from build123d import *

# Parameters (mm, degrees)
SKETCH1_W           = 400
SKETCH1_H           = 80
BOSS_EXTRUDE1_DEPTH = 20
SKETCH5_W           = 400
SKETCH5_H           = 10
BOSS_EXTRUDE2_DEPTH = 30
SKETCH7_W           = 400
SKETCH7_H           = 10
BOSS_EXTRUDE3_DEPTH = 30
BOSS_EXTRUDE4_START = -20
SKETCH8_W           = 100
SKETCH8_H           = 60
BOSS_EXTRUDE4_DEPTH = 490
SKETCH9_W           = 80
SKETCH9_H           = 50
CUT_EXTRUDE1_DEPTH  = 940
SKETCH11_W          = 80
SKETCH11_H          = 50
BOSS_EXTRUDE5_DEPTH = 20
MIRROR20_START      = -30
MIRROR20_OUTLINE_W  = 490
MIRROR20_OUTLINE_H  = 100
MIRROR20_DEPTH      = 60
SKETCH12_R          = 15
CUT_EXTRUDE2_DEPTH  = 1031.388276331
SKETCH19_R          = 15
CUT_EXTRUDE10_DEPTH = 1031.388276331


# Read off the part's stored shape, not the designer's step: Mirror20
with BuildPart() as part:
    # Sketch1 → Boss-Extrude1 (new body)
    with BuildSketch(Plane(origin=(0, 0, 0), x_dir=(0, 0, -1), z_dir=(1, 0, 0))):
        Rectangle(SKETCH1_W, SKETCH1_H)
    boss_extrude1 = extrude(amount=BOSS_EXTRUDE1_DEPTH)

    # Sketch5 → Boss-Extrude2 (add)
    with BuildSketch(Plane.ZY):
        with Locations((0, 35)):
            Rectangle(SKETCH5_W, SKETCH5_H)
    boss_extrude2 = extrude(amount=BOSS_EXTRUDE2_DEPTH)

    # Sketch7 → Boss-Extrude3 (add)
    with BuildSketch(Plane(origin=(20, 0, 0), x_dir=(0, 0, -1), z_dir=(1, 0, 0))):
        with Locations((0, -35)):
            Rectangle(SKETCH7_W, SKETCH7_H)
    boss_extrude3 = extrude(amount=BOSS_EXTRUDE3_DEPTH)

    # Sketch8 → Boss-Extrude4 (add)
    with BuildSketch(Plane.ZY.offset(BOSS_EXTRUDE4_START)):
        Rectangle(SKETCH8_W, SKETCH8_H)
    extrude(amount=BOSS_EXTRUDE4_DEPTH)

    # Sketch9 → Cut-Extrude1 (cut)
    with BuildSketch(Plane.ZY.offset(470)):
        with Locations((0, -5)):
            Rectangle(SKETCH9_W, SKETCH9_H)
    cut_extrude1 = extrude(amount=-CUT_EXTRUDE1_DEPTH, mode=Mode.SUBTRACT)

    # Sketch11 → Boss-Extrude5 (add)
    with BuildSketch(Plane(origin=(20, 0, 0), x_dir=(0, 0, -1), z_dir=(1, 0, 0))):
        with Locations((0, -5)):
            Rectangle(SKETCH11_W, SKETCH11_H)
    boss_extrude5 = extrude(amount=-BOSS_EXTRUDE5_DEPTH)

    # Mirror20 outline → Mirror20 (add)
    with BuildSketch(Plane(origin=(0, 0, 0), x_dir=(1, 0, 0), z_dir=(0, 1, 0)).offset(MIRROR20_START)):
        with Locations((-715, 0)):
            Rectangle(MIRROR20_OUTLINE_W, MIRROR20_OUTLINE_H)
    extrude(amount=MIRROR20_DEPTH)

    # Mirror22: Boss-Extrude1, Boss-Extrude2, Boss-Extrude3, Cut-Extrude1, Boss-Extrude5 across plane
    add(boss_extrude1.mirror(Plane.ZY.offset(470)))
    add(boss_extrude2.mirror(Plane.ZY.offset(470)))
    add(boss_extrude3.mirror(Plane.ZY.offset(470)))
    add(cut_extrude1.mirror(Plane.ZY.offset(470)), mode=Mode.SUBTRACT)
    add(boss_extrude5.mirror(Plane.ZY.offset(470)))

    # Sketch12 → Cut-Extrude2 (cut, through all)
    with BuildSketch(Plane.ZY.offset(960)):
        with Locations((89.62, 0)):
            Circle(SKETCH12_R)
    extrude(amount=-CUT_EXTRUDE2_DEPTH, mode=Mode.SUBTRACT)

    # Sketch19 → Cut-Extrude10 (cut, through all)
    with BuildSketch(Plane.ZY.offset(960)):
        with Locations((-128.216, 0)):
            Circle(SKETCH19_R)
    extrude(amount=-CUT_EXTRUDE10_DEPTH, mode=Mode.SUBTRACT)


solid = part.part
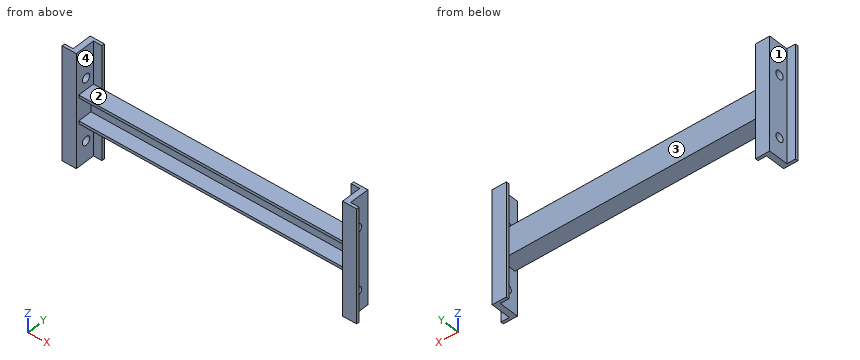
Work out the finished part from the listing and answer in its coordinate system (mm). Face numbers are marked on the shaded views. A direction names the side the tool comes from. Give positions to 0.01 mm unless a question says otherwise; leave off trailing zeros. Loops run counter-clockwise (first coordinate to the right, second up) from the corner with the lowest first, then second, coordinate; pieces in that order, holes last. Notation, with made-up numbers: (22.25, 53.5) -> (49.25, 53.5) arc R17 cw to (49.25, 72.5) -> close; hole circle Ø4 at (7, 52.25). An arc over 180 degrees is marked (long way). Use a Markdown table: item, result. Add a question column.
1. Flat-ended cylindrical pins translate along their axes: pin 1 Ø15 at (x, z) = (-977.5, -50) entering from +Y; pin 2 Ø2 at (y, z) = (-27, -24) entering from +X; pin 3 Ø4 at (x, z) = (-586.5, -47) entering from -Y; pin 4 Ø24 at (y, z) = (0, -128.216) entering from +X (3 decimals). Find the tip coordinate at first contact, or state that the pin passes through.
2. For the marked faces 3 and 4, determine the directions among +Z, -Z, +X, -X, +Y, -Y from which every point of the face is accessible in a straight line to the end or side of a thin tool.
3. Section C-C on x = -456 is taken. Determine the outline of the cut face in (y, z), and give its area (3 significant figures).
4. Find the intervals of material crossed by probe 1 along X at (y, z) = (-26, 67); probe 2 along X at (y, z) = (-30.5, -42); probe 3 along Z at (x, y) = (-23, 4), in increasing order.
5. Determine the mould class of the marked faces 1 and 2 for opening direction X: released by +X, released by -X, zero draft, split by the parting line, or undercut.
6. Section D-D on z = -22 is taken. Determine the outline of the cut face in (x, y), and give its area (3 significant figures).
7. Section B-B on z = -125 is taken. Determine the outline of the cut face in (x, y), and give its area (3 significant figures).
8. Section A-A on y = 0 is taken. State how many separate pieces and enclosed holes the cut face has, and give its area (3 significant figures).
Results below:
| question | item | result |
|---|---|---|
| 1 | pin 1 | stops at y = -30 |
| 1 | pin 2 | stops at x = 20 |
| 1 | pin 3 | stops at y = -30 |
| 1 | pin 4 | passes through |
| 2 | face 3 | +Z, -Z, +Y |
| 2 | face 4 | -Y |
| 3 | outline | (-30, -50) -> (30, -50) -> (30, 50) -> (-30, 50) -> (-30, 40) -> (20, 40) -> (20, -40) -> (-30, -40) -> close |
| 3 | area | 2,000 mm^2 |
| 4 | probe 1 | x = -960 to -940, 0 to 20 |
| 4 | probe 2 | x = -990 to -940, 0 to 50 |
| 4 | probe 3 | z = -50 to -40, 40 to 50 |
| 5 | face 1 | released by -X |
| 5 | face 2 | undercut |
| 6 | outline | (-990, -40) -> (-940, -40) -> (-940, 20) -> (0, 20) -> (0, -40) -> (50, -40) -> (50, -30) -> (20, -30) -> (20, 40) -> (-30, 40) -> (-30, 30) -> (-910, 30) -> (-910, 40) -> (-960, 40) -> (-960, -30) -> (-990, -30) -> close |
| 6 | area | 13,800 mm^2 |
| 7 | outline | (-990, -40) -> (-940, -40) -> (-940, -14.65) -> (-960, -14.65) -> (-960, -30) -> (-990, -30) -> close; (-960, 14.65) -> (-940, 14.65) -> (-940, 30) -> (-910, 30) -> (-910, 40) -> (-960, 40) -> close; (-30, 30) -> (0, 30) -> (0, 14.65) -> (20, 14.65) -> (20, 40) -> (-30, 40) -> close; (0, -40) -> (50, -40) -> (50, -30) -> (20, -30) -> (20, -14.65) -> (0, -14.65) -> close |
| 7 | area | 3,230 mm^2 |
| 8 | separate pieces | 5 |
| 8 | enclosed holes | 1 |
| 8 | area | 32,400 mm^2 |
